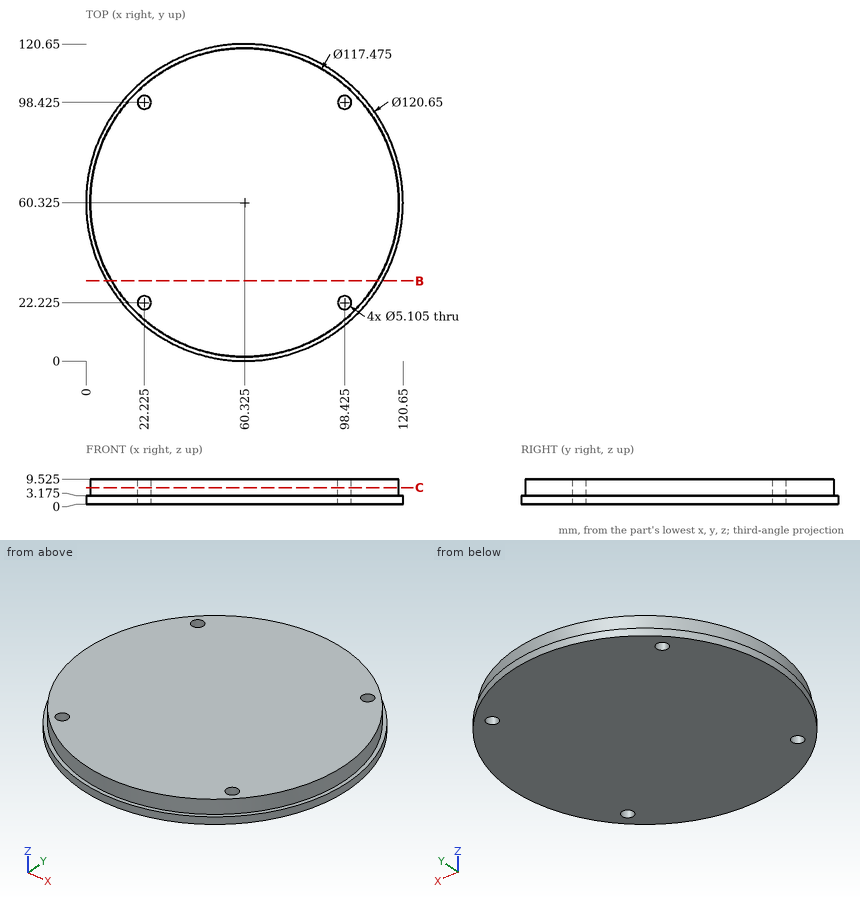
Source: three-view drawing plus pictorial views. Frame: mm from the lowest corner of the part. Coordinates: 2 decimals unless noted, no trailing zeros. Loops run counter-clockwise (first coordinate to the right, second up) from the corner with the lowest first, then second, coordinate; pieces in that order, holes last. Notation, with made-up numbers: M 54,17.5 L 97,17.5 A25 cw 97,51.5 Z; hole C -17.5,50 d11. An arc over 180 degrees is marked long. Use CSV: the item, a comma, the result in double quotes.
(1) Cut plane B-B on y = 30.5. Return loops of the section in (x, z) (1 decimal).
Answers follow:
outline,"M 7.9,0 L 112.8,0 L 112.8,3.2 L 110.9,3.2 L 110.9,9.5 L 9.7,9.5 L 9.7,3.2 L 7.9,3.2 Z"
(2) Contact query for flat-ended pins moving along their axis: pin 1 (4 mm diameter, centred on x = 98.425, y = 22.225, fed in from +Z); pin 2 (3 mm diameter, centred on x = 55.5, z = 3, fed in from +Y); pin 3 (5 mm diameter, centred on y = 69.5, z = 6, fed in from -X); pin 4 (5 mm diameter, centred on y = 21.5, z = 4, fed in from +X). Output: stop coordinate, or through.
Answers follow:
pin 1,"through"
pin 2,"y = 120.56"
pin 3,"x = 1.97"
pin 4,"x = 108.38"
(3) Cut plane C-C on z = 6.25. Return loops of the section in (x, y) (1 decimal), and give its area (3 significant figures).
Answers follow:
outline,"C 60.3,60.3 d117.5; hole C 22.2,22.2 d5.1; hole C 22.2,98.4 d5.1; hole C 98.4,22.2 d5.1; hole C 98.4,98.4 d5.1"
area,"10,800 mm²"
(4) Line query: line 1 (X direction, y = 99.5, z = 0.75); line 2 (X direction, y = 62, z = 5.75); line 3 (Y direction, x = 112, z = 4). Output: solid intervals per line, ascending. Write a range as [from, to].
Answers follow:
line 1,"[14.45, 19.91], [24.54, 96.11], [100.74, 106.2]"
line 2,"[1.61, 119.04]"
line 3,"[32.4, 88.25]"
